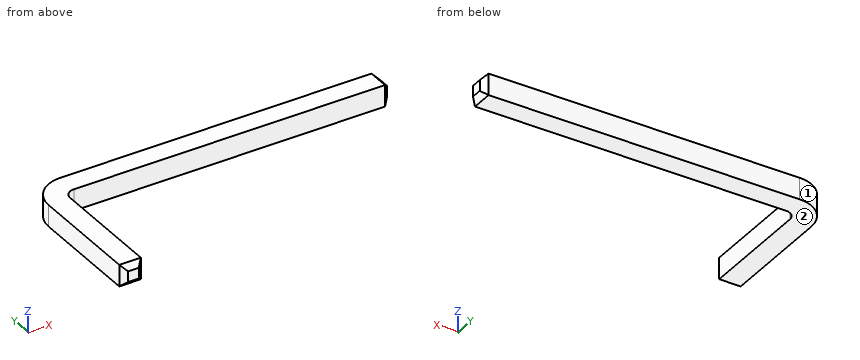
```python
from build123d import *

# Parameters (mm, degrees)
BODY_DEPTH     = 0.65
CHAMFER_2_SIZE = 0.1625


with BuildPart() as part:
    # Sketch1 → Body (new body)
    with BuildSketch(Plane.XY):
        with BuildLine():
            Line((0, 3.55), (0, 0))
            Line((0, 0), (0.65, 0))
            Line((0.65, 0), (0.65, 3.55))
            ThreePointArc((0.65, 3.55), (0.737867966, 3.762132034), (0.95, 3.85))
            Line((0.95, 3.85), (10.5, 3.85))
            Line((10.5, 3.85), (10.5, 4.5))
            Line((10.5, 4.5), (0.95, 4.5))
            ThreePointArc((0.95, 4.5), (0.278248558, 4.221751442), (0, 3.55))
        make_face()
    extrude(amount=BODY_DEPTH)

    # Chamfer 2
    chamfer_2_edges = [part.edges().sort_by_distance(p)[0] for p in [
        (0, 0, 0.325),
        (0.65, 0, 0.325),
        (0.325, 0, 0),
        (0.325, 0, 0.65),
        (10.5, 3.85, 0.325),
        (10.5, 4.5, 0.325),
        (10.5, 4.175, 0),
        (10.5, 4.175, 0.65),
    ]]
    chamfer(chamfer_2_edges, length=CHAMFER_2_SIZE)


solid = part.part
```
Work out the finished part from the listing and answer in its coordinate system (mm). Face numbers are marked on the shaded views. Give positions to 0.01 mm unless a question says otherwise; leave off trailing zeros. Loops run counter-clockwise (first coordinate to the right, second up) from the corner with the lowest first, then second, coordinate; pieces in that order, holes last. Notation, with made-up numbers: M 75,24 L 112,24 A32 cw 112,62 Z; hole C 33,-15 d3. An arc over 180 degrees is marked long. One line per item, written item: value. Start each with the question number.
1. Find section B-B (x = 9.5). Give the vertices of the cut face in (y, z), and give its area (4 significant figures).
2. Determine the mould class of the marked faces 1 and 2 for opening direction X: released by +X, released by -X, zero draft, split by the parting line, or undercut.
3. Find section A-A (z = 0.3). Give the vertices of the cut face in (x, y).
4. Find the intervals of material crossed by probe 1 along X at (y, z) = (0.2, 0.2); probe 2 along Y at (x, z) = (3.5, 0.2); probe 3 along X at (y, z) = (3.9, 0.4), in increasing order.
5. Find section C-C (y = 0.6). Give the vertices of the cut face in (x, z), and give its area (4 significant figures).
6. This flat-tipped pin is pushed along its axis until it touches: P1, Ø1, axis at x = 8, y = 3.5, coming from the -Z side. Where does it stop, or does it pass through?
Reported:
1. outline: M 3.85,0 L 4.5,0 L 4.5,0.65 L 3.85,0.65 Z
1. area: 0.4225 mm²
2. face 1: released by -X
2. face 2: zero draft
3. outline: M 0,0.16 L 0.16,0 L 0.49,0 L 0.65,0.16 L 0.65,3.55 A0.3 cw 0.95,3.85 L 10.34,3.85 L 10.5,4.01 L 10.5,4.34 L 10.34,4.5 L 0.95,4.5 A0.95 ccw 0,3.55 Z
4. probe 1: x = 0 to 0.65
4. probe 2: y = 3.85 to 4.5
4. probe 3: x = 0.07 to 10.39
5. outline: M 0,0 L 0.65,0 L 0.65,0.65 L 0,0.65 Z
5. area: 0.4225 mm²
6. P1: stops at z = 0
